Design review of the part built by this model. Coordinates are the model's own, in mm. Face numbers are marked on the shaded views. Give positions to 0.01 mm unless a question says otherwise; leave off trailing zeros. Loops run counter-clockwise (first coordinate to the right, second up) from the corner with the lowest first, then second, coordinate; pieces in that order, holes last. Notation, with made-up numbers: (18.5, 71) -> (30.5, 71) arc R33 ccw to (30.5, 99) -> close; hole circle Ø10 at (37, 59). An arc over 180 degrees is marked (long way). Answer in a Markdown table with one row per item. Add a question column.
(1) Consider section A-A on x = -88. Write out the cut boundary in (y, z).
(2) Consider section C-C on y = -176.5. Write out the cut boundary in (x, z), then the cut area to 3 significant figures.
(3) Draft analysis for pull direction Y (two halves, no side actions). For the marked faces 1, 2 and 3, state which applies: +Y half, -Y half, draft (parallel to the pull), parting line (faces both ways), or undercut.
(4) For line 1 (Y direction, x = 94.5, z = 455.5); line 2 (X direction, y = 219.5, z = 1150.5); line 3 (Y direction, x = 22.5, z = 189), list the stretches that pass through material, from the lowest coordinate up.
(5) Consider section B-B on z = 968. Write out the cut boundary in (x, y), then the cut area to 3 significant figures.
(6) For pin 1 (10 mm diameter, centred on y = -170, z = 1360, fed in from +X); pin 2 (10 mm diameter, centred on y = 235.5, z = 1838, fed in from -X), all flat-tipped, find the tip position at first contact; note any pin that passes through.
Autodesk Inventor part; units mm, degrees
ref_plane "Start plane" through (0, 0, 0) normal (0, 0, 1) x (1, 0, 0)
ref_plane "End plane" through (0, 0, 2100) normal (0, 0, 1) x (1, 0, 0)
ref_plane "YZ Plane" through (0, 0, 0) normal (1, 0, 0) x (0, 1, 0)
ref_plane "Start plane" through (0, 0, 0) normal (0, 0, 1) x (1, 0, 0)
ref_plane "End plane" through (0, 0, 2100) normal (0, 0, 1) x (1, 0, 0)
sketch "Sketch" plane through (0, 0, 0) normal (0, 0, 1) x (1, 0, 0)
  line L0 (-136, -390.5) -> (-136, -359.2)
  line L1 (-136, -359.2) -> (-26.15, -359.2)
  line L2 (-9.65, -342.7) -> (-9.65, 0)
  line L3 (-9.65, 0) -> (0, 0) construction
  line L4 (0, 0) -> (0, -390.5) construction
  line L5 (0, -390.5) -> (-136, -390.5)
  line L6 (-60, 0) -> (80, 0) construction
  line L7 (0, -60) -> (0, 80) construction
  line L8 (136, -390.5) -> (136, -359.2)
  line L9 (136, -359.2) -> (26.15, -359.2)
  line L10 (9.65, -342.7) -> (9.65, 0)
  line L11 (9.65, 0) -> (0, 0) construction
  line L12 (0, -390.5) -> (136, -390.5)
  line L13 (-136, 390.5) -> (-136, 359.2)
  line L14 (-136, 359.2) -> (-26.15, 359.2)
  line L15 (-9.65, 342.7) -> (-9.65, 0)
  line L16 (0, 390.5) -> (-136, 390.5)
  line L17 (136, 390.5) -> (136, 359.2)
  line L18 (136, 359.2) -> (26.15, 359.2)
  line L19 (0, 390.5) -> (136, 390.5)
  line L20 (9.65, 342.7) -> (9.65, 0)
  arc A0 (-9.65, 342.7) -> (-26.15, 359.2) centre (-26.15, 342.7) ccw
  arc A1 (26.15, 359.2) -> (9.65, 342.7) centre (26.15, 342.7) ccw
  arc A2 (9.65, -342.7) -> (26.15, -359.2) centre (26.15, -342.7) ccw
  arc A3 (-26.15, -359.2) -> (-9.65, -342.7) centre (-26.15, -342.7) ccw
  line L21 (0, 108) -> (0, -88) construction
  line L22 (-88, 0) -> (108, 0) construction
  point P0 (-9.65, -359.2)
  point P1 (9.65, -359.2)
  point P2 (-9.65, 359.2)
  point P3 (9.65, 359.2)
  dimension "d1" = 390.5
  dimension "d2" = 31.3
  dimension "d3" = 136
  dimension "d4" = 9.65
  dimension "d10" = 16.5
extrude "Body" add sketch "Sketch" along normal up to surface (2100 mm away) from surface at 0
sketch "Sketch4" plane through (0, 0, 0) normal (0, 0, 1) x (1, 0, 0)
  line L0 (0, 0) -> (10, 0)
ref_plane "Work Plane3" through (0, 0, 0) normal (0, -1, 0) x (1, 0, 0)
sketch "Sketch5" plane through (0, 0, 0) normal (0, -1, 0) x (1, 0, 0)
  line L0 (-2, 0) -> (12, 0)
  line L1 (-2, 2100) -> (12, 2100)
  dimension "d14" = 2100
equation "\"d1\" = 0.5 * G_H"
equation "\"d2\" = G_T1"
equation "\"d3\" = 0.5 * G_W"
equation "\"d4\" = 0.5 * G_T"
equation "\"d10\" = G_IR"
equation "\"d5\" = G_L"
equation "\"G_W\" = 272"
equation "\"G_H\" = 781"
equation "\"G_T\" = 19.3"
equation "\"G_T1\" = 31.3"
equation "\"G_IR\" = 16.5"
equation "\"G_L\" = d14"
equation "\"G_OFFSET_START\" = 0"
equation "\"G_OFFSET_END\" = 0"
properties part number "AS 3679-1990 - 760 UB - 244 - 2100" material "Steel, Mild"
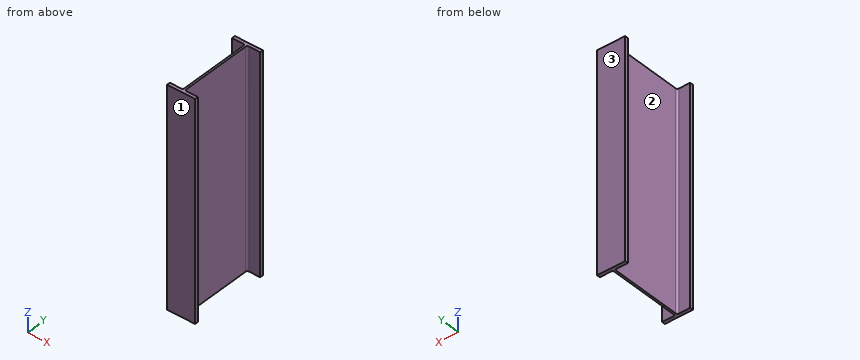
Values follow:
| question | item | result |
|---|---|---|
| 1 | outline | (-390.5, 0) -> (-359.2, 0) -> (-359.2, 2100) -> (-390.5, 2100) -> close; (359.2, 0) -> (390.5, 0) -> (390.5, 2100) -> (359.2, 2100) -> close |
| 2 | outline | (-9.65, 0) -> (9.65, 0) -> (9.65, 2100) -> (-9.65, 2100) -> close |
| 2 | area | 40,500 mm2 |
| 3 | face 1 | -Y half |
| 3 | face 2 | undercut |
| 3 | face 3 | +Y half |
| 4 | line 1 | -390.5 to -359.2, 359.2 to 390.5 |
| 4 | line 2 | -9.65 to 9.65 |
| 4 | line 3 | -390.5 to -358.79, 358.79 to 390.5 |
| 5 | outline | (-136, -390.5) -> (136, -390.5) -> (136, -359.2) -> (26.15, -359.2) arc R16.5 cw to (9.65, -342.7) -> (9.65, 342.7) arc R16.5 cw to (26.15, 359.2) -> (136, 359.2) -> (136, 390.5) -> (-136, 390.5) -> (-136, 359.2) -> (-26.15, 359.2) arc R16.5 cw to (-9.65, 342.7) -> (-9.65, -342.7) arc R16.5 cw to (-26.15, -359.2) -> (-136, -359.2) -> close |
| 5 | area | 31,100 mm2 |
| 6 | pin 1 | x = 9.65 |
| 6 | pin 2 | x = -9.65 |
